Could you check a few things on this model? Use its own coordinates, in mm. Give positions to 0.01 mm unless a question says otherwise; leave off trailing zeros. Loops run counter-clockwise (first coordinate to the right, second up) from the corner with the lowest first, then second, coordinate; pieces in that order, holes last.
1. Imagine slicing it at A-A (y = -126.5). List the corners of the cut face in (x, z) for me.
2. I need wall thicknesses on line 1 along Y through (x, z) = (-89.5, 2.8); line 2 along X through (y, z) = (-70, 2.85); line 3 along Y through (x, z) = (47.5, 2.5). Which ranges of each line are inside material? Lowest first, please.
3. For P1, Ø1, axis at x = 132, z = 2.5, coming from the -Y side; P2, Ø1.6, axis at x = 134.5, z = 2.5, coming from the -Y side; P3, Ø3, axis at x = 218, y = -70, coming from the -Z side; P4, Ø1.2, axis at y = -117, z = 1.5, coming from the +X side, each with a flat end and sliding along its axis, tell me the tip position at first contact or that it passes through.
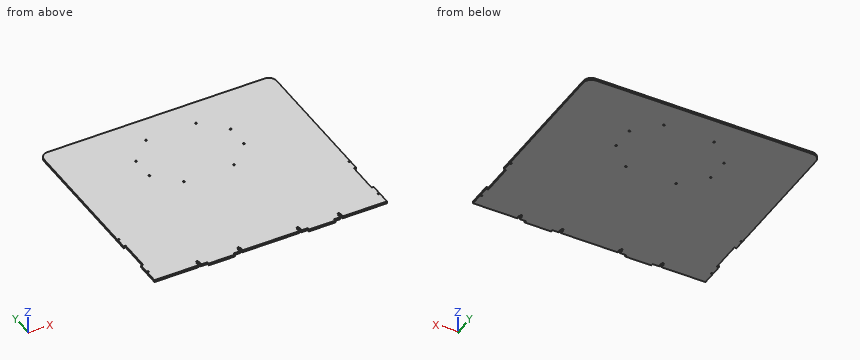
```python
from build123d import *

# Parameters (mm, degrees)
ESQUISSE1_W             = 440
ESQUISSE1_H             = 390
BOSS_EXTRU_1_DEPTH      = 4
ESQUISSE2_W             = 50
ESQUISSE2_H             = 4
BOSS_EXTRU_2_DEPTH      = 4
ESQUISSE3_W             = 4
ESQUISSE3_H             = 60
ENL_V_MAT_EXTRU_1_DEPTH = 4
CONG_1_R                = 15
ESQUISSE4_R             = 1.6
ENL_V_MAT_EXTRU_2_DEPTH = 10
ESQUISSE5_R             = 1.6
ENL_V_MAT_EXTRU_3_DEPTH = 4


with BuildPart() as part:
    # Esquisse1 → Boss.-Extru.1 (new body)
    with BuildSketch(Plane.XY):
        Rectangle(ESQUISSE1_W, ESQUISSE1_H)
    extrude(amount=BOSS_EXTRU_1_DEPTH)

    # Esquisse2 → Boss.-Extru.2 (add)
    with BuildSketch(Plane(origin=(0, 0, 0), x_dir=(-1, 0, 0), z_dir=(0, 0, -1))):
        with Locations((-95, -197)):
            Rectangle(ESQUISSE2_W, ESQUISSE2_H)
        with Locations((95, -197)):
            Rectangle(ESQUISSE2_W, ESQUISSE2_H)
    extrude(amount=-BOSS_EXTRU_2_DEPTH)

    # Esquisse3 → Enlèv. mat.-Extru.1 (cut)
    with BuildSketch(Plane(origin=(0, 0, 0), x_dir=(-1, 0, 0), z_dir=(0, 0, -1))):
        with Locations((-218, -120)):
            Rectangle(ESQUISSE3_W, ESQUISSE3_H)
        with Locations((218, -120)):
            Rectangle(ESQUISSE3_W, ESQUISSE3_H)
    extrude(amount=-ENL_V_MAT_EXTRU_1_DEPTH, mode=Mode.SUBTRACT)

    # Congé1
    cong_1_edges = [part.edges().sort_by_distance(p)[0] for p in [
        (-220, 195, 2),
        (220, 195, 2),
    ]]
    fillet(cong_1_edges, radius=CONG_1_R)

    # Esquisse4 → Enlèv. mat.-Extru.2 (cut)
    with BuildSketch(Plane(origin=(0, 0, 0), x_dir=(-1, 0, 0), z_dir=(0, 0, -1))):
        Polygon((-132.4, -195), (-132.4, -192), (-131.15, -192), (-131.15, -187.8), (-132.4, -187.8), (-132.4, -184), (-135.6, -184), (-135.6, -187.8), (-136.85, -187.8), (-136.85, -192), (-135.6, -192), (-135.6, -195), align=None)
        Polygon((-57.6, -192), (-57.6, -195), (-54.4, -195), (-54.4, -192), (-53.15, -192), (-53.15, -187.8), (-54.4, -187.8), (-54.4, -184), (-57.6, -184), (-57.6, -187.8), (-58.85, -187.8), (-58.85, -192), align=None)
        with Locations((-218, -170)):
            Circle(ESQUISSE4_R)
        with Locations((-218, -70)):
            Circle(ESQUISSE4_R)
        with Locations((218, -70)):
            Circle(ESQUISSE4_R)
        with Locations((218, -170)):
            Circle(ESQUISSE4_R)
        Polygon((54.4, -192), (54.4, -195), (57.6, -195), (57.6, -192), (58.85, -192), (58.85, -187.8), (57.6, -187.8), (57.6, -184), (54.4, -184), (54.4, -187.8), (53.15, -187.8), (53.15, -192), align=None)
        Polygon((135.6, -187.8), (135.6, -184), (132.4, -184), (132.4, -187.8), (131.15, -187.8), (131.15, -192), (132.4, -192), (132.4, -195), (135.6, -195), (135.6, -192), (136.85, -192), (136.85, -187.8), align=None)
    extrude(amount=-ENL_V_MAT_EXTRU_2_DEPTH, mode=Mode.SUBTRACT)

    # Esquisse5 → Enlèv. mat.-Extru.3 (cut)
    with BuildSketch(Plane(origin=(0, 0, 0), x_dir=(-1, 0, 0), z_dir=(0, 0, -1))):
        with Locations((-47.5, 144.040872052)):
            Circle(ESQUISSE5_R)
        with Locations((-89.5, 102.040872052)):
            Circle(ESQUISSE5_R)
        with Locations((-89.5, 57.040872052)):
            Circle(ESQUISSE5_R)
        with Locations((-47.5, 15.040872052)):
            Circle(ESQUISSE5_R)
        with Locations((89.5, 57.040872052)):
            Circle(ESQUISSE5_R)
        with Locations((47.5, 15.040872052)):
            Circle(ESQUISSE5_R)
        with Locations((47.5, 144.040872052)):
            Circle(ESQUISSE5_R)
        with Locations((89.5, 102.040872052)):
            Circle(ESQUISSE5_R)
    extrude(amount=-ENL_V_MAT_EXTRU_3_DEPTH, mode=Mode.SUBTRACT)


solid = part.part
```
Derived:
1. outline: (-216, 0) - (216, 0) - (216, 4) - (-216, 4) - close
2. line 1: y = -199 to 55.44, 58.64 to 100.44, 103.64 to 195
2. line 2: x = -220 to -219.6, -216.4 to 216.4, 219.6 to 220
2. line 3: y = -195 to 13.44, 16.64 to 142.44, 145.64 to 195
3. P1: stops at y = -195
3. P2: stops at y = -184
3. P3: passes through
3. P4: stops at x = 216
